Autodesk Fusion 360 part; units mm, degrees
sketch "Sketch1" plane through (0, 0, 0) normal (0, 1, 0) x (1, 0, 0) in component "Raam_v3"
  line L0 (-100, 100) -> (100, 100)
  line L1 (100, 100) -> (100, -100)
  line L2 (100, -100) -> (-100, -100)
  line L3 (-100, -100) -> (-100, 100)
  circle A0 centre (0, 0) radius 82.5
  line L4 (-70.5, -70.5) -> (70.5, -70.5) construction
  line L5 (70.5, -70.5) -> (70.5, 70.5) construction
  line L6 (70.5, 70.5) -> (-70.5, 70.5) construction
  line L7 (-70.5, 70.5) -> (-70.5, -70.5) construction
  line L8 (-46, -100) -> (46, -100)
  line L9 (46, -100) -> (46, -68)
  line L10 (46, -68) -> (-46, -68)
  line L11 (-46, -68) -> (-46, -100)
  line L12 (-46, 100) -> (46, 100)
  line L13 (46, 100) -> (46, 68)
  line L14 (46, 68) -> (-46, 68)
  line L15 (-46, 68) -> (-46, 100)
  circle A1 centre (70.5, -70.5) radius 5
  circle A2 centre (-70.5, -70.5) radius 5
  circle A3 centre (70.5, 70.5) radius 5
  circle A4 centre (-70.5, 70.5) radius 5
  line L16 (-91.25, -91.25) -> (91.25, -91.25) construction
  line L17 (91.25, -91.25) -> (91.25, 91.25) construction
  line L18 (91.25, 91.25) -> (-91.25, 91.25) construction
  line L19 (-91.25, 91.25) -> (-91.25, -91.25) construction
  line L20 (0, -100) -> (0, 100) construction
  line L21 (-100, 0) -> (100, 0) construction
  line L22 (-100, -75) -> (-74.4285, -100)
  line L23 (100, -75) -> (75.5588, -100)
  line L24 (-100, 75) -> (-75.5588, 100)
  line L25 (74.4285, 100) -> (100, 75)
  circle A5 centre (-91.25, 0) radius 1.5
  circle A6 centre (91.25, 0) radius 1.5
  line L26 (-100, -75) -> (100, -75) construction
  circle A7 centre (91.25, -75) radius 1.5
  line L27 (-100, 75) -> (100, 75) construction
  circle A8 centre (91.25, 75) radius 1.5
  circle A9 centre (-91.25, 75) radius 1.5
  circle A10 centre (-91.25, -75) radius 1.5
  line L28 (-95.1383, -79.753) -> (-77.6201, -79.753)
  line L29 (-77.6201, -79.753) -> (-77.6201, -96.8797)
  line L30 (-83.7274, -79.753) -> (-83.7274, -80)
  line L31 (95.3116, -79.7956) -> (78.4368, -79.7956)
  line L32 (78.4368, -79.7956) -> (78.4368, -97.0562)
  line L33 (-95.1178, 79.9938) -> (-80.1166, 79.9938)
  line L34 (-80.1166, 79.9938) -> (-80.1166, 95.3379)
  line L35 (94.9708, 79.9168) -> (79.5428, 79.9168)
  line L36 (79.5428, 79.9168) -> (79.5428, 95)
  dimension "d1" = 200
  dimension "d2" = 200
  dimension "d3" = 165
  dimension "d6" = 141
  dimension "d7" = 141
  dimension "d8" = 29.5
  dimension "d9" = 29.5
  dimension "d11" = 100
  dimension "d12" = 100
  dimension "d18" = 92
  dimension "d19" = 32
  dimension "d20" = 46
  dimension "d21" = 92
  dimension "d22" = 32
  dimension "d23" = 46
  dimension "d24" = 10
  dimension "d25" = 10
  dimension "d26" = 10
  dimension "d27" = 10
  dimension "d28" = 182.5
  dimension "d29" = 182.5
  dimension "d30" = 70.5
  dimension "d31" = 8.75
  dimension "d32" = 8.75
  dimension "d33" = 3
  dimension "d34" = 3
  dimension "d53" = 12.3744
  dimension "d54" = 12.3744
  dimension "d55" = 12.3744
  dimension "d56" = 12.3744
  dimension "d57" = 41.7193
  dimension "d58" = 41.7193
  dimension "d59" = 75
  dimension "d60" = 3
  dimension "d61" = 75
  dimension "d62" = 3
  dimension "d63" = 3
  dimension "d64" = 3
extrude "Extrude11" add sketch "Sketch1" along normal blind 1.25 contours L0 A0 L12 L13 L15 | L2 A0 L8 L9 L11 makes body 1 at (0, 0, -94.1667) makes body 2 at (0, 0, 94.1667) in component "Raam_v3"
extrude "Extrude10" add sketch "Sketch1" along normal blind 2 separate body contours L0 L2 L3 A0 L11 L15 L22 L24 L28 L29 L33 L34 | L0 L1 L2 A0 L9 L13 L23 L25 L31 L32 L35 L36 makes body 3 at (-63.4107, 0, -91.7181) makes body 4 at (63.4107, 2, 91.7181) in component "Raam_v3"
extrude "Extrude12" add sketch "Sketch1" along normal blind 3.5 contours A2 bodies 3 in component "Raam_v3"
extrude "Extrude13" add sketch "Sketch1" along normal blind 3.5 contours A1 bodies 4 in component "Raam_v3"
extrude "Extrude14" add sketch "Sketch1" along normal blind 3.5 contours A4 bodies 3 in component "Raam_v3"
extrude "Extrude15" add sketch "Sketch1" along normal blind 3.5 contours A3 bodies 4 in component "Raam_v3"
extrude "Extrude16" add 1 faces at (63.4107, 2, 91.7181) along direction (0, 1, 0) blind 2 on bodies 4 bodies 4 in component "Raam_v3"
extrude "Extrude17" add 1 faces at (-63.4107, 2, -91.7181) along direction (0, 1, 0) blind 2 on bodies 3 bodies 3 in component "Raam_v3"
extrude "Extrude18" add 1 faces at (0, 1.25, 94.1667) along direction (0, 1, 0) blind 1 on bodies 2 bodies 2 3 4 in component "Raam_v3"
extrude "Extrude19" add 1 faces at (0, 1.25, -94.1667) along direction (0, 1, 0) blind 1 on bodies 1 bodies 1 2 in component "Raam_v3"
extrude "Extrude20" add 1 faces at (-69.0538, 3.5, 70.0197) along direction (0, 1, 0) blind 4 on bodies 1 bodies 1 in component "Raam_v3"
extrude "Extrude21" cut 1 faces at (-69.0538, 7.5, 70.0197) along direction (0, -1, 0) blind 1 on bodies 1 bodies 1 in component "Raam_v3"
extrude "Extrude22" add 1 faces at (71.8216, 3.5, 69.804) along direction (0, 1, 0) blind 3 on bodies 1 bodies 1 in component "Raam_v3"
extrude "Extrude23" add 1 faces at (-69.0538, 3.5, -70.9803) along direction (0, 1, 0) blind 3 on bodies 1 bodies 1 in component "Raam_v3"
extrude "Extrude24" cut 1 faces at (-63.4107, 4, -91.7181) along direction (0, -1, 0) blind 1 on bodies 1 bodies 1 in component "Raam_v3"
extrude "Extrude25" cut 1 faces at (63.4107, 4, 91.7181) along direction (0, -1, 0) blind 1 on bodies 1 bodies 1 in component "Raam_v3"
extrude "Extrude26" cut 1 faces at (0, 2.25, 94.1667) along direction (0, -1, 0) blind 0.5 on bodies 1 bodies 1 in component "Raam_v3"
extrude "Extrude27" cut 1 faces at (0, 2.25, -94.1667) along direction (0, -1, 0) blind 0.5 on bodies 1 bodies 1 in component "Raam_v3"
extrude "Extrude28" cut 1 faces at (-69.0538, 6.5, 70.0197) along direction (0, -1, 0) blind 1 on bodies 1 bodies 1 in component "Raam_v3"
extrude "Extrude29" cut 1 faces at (71.8216, 6.5, 69.804) along direction (0, -1, 0) blind 1 on bodies 1 bodies 1 in component "Raam_v3"
extrude "Extrude30" cut 1 faces at (71.8216, 3.5, -71.196) along direction (0, -1, 0) blind 1 on bodies 1 bodies 1 in component "Raam_v3"
extrude "Extrude31" cut 1 faces at (-69.0538, 6.5, -70.9803) along direction (0, -1, 0) blind 1 on bodies 1 bodies 1 in component "Raam_v3"
extrude "Extrude32" add 1 faces at (71.8216, 2.5, -71.196) along direction (0, 1, 0) blind 3 on bodies 1 bodies 1 in component "Raam_v3"
extrude "Extrude2" [suppressed] in component "Raam_v3"
extrude "Extrude1" [suppressed] in component "Raam_v3"
extrude "Extrude3" [suppressed] in component "Raam_v3"
extrude "Extrude4" [suppressed] in component "Raam_v3"
extrude "Extrude5" [suppressed] in component "Raam_v3"
extrude "Extrude6" [suppressed] in component "Raam_v3"
extrude "Extrude7" [suppressed] in component "Raam_v3"
extrude "Extrude8" [suppressed] in component "Raam_v3"
extrude "Extrude9" [suppressed] in component "Raam_v3"
hole "Hole1" [suppressed] in component "Raam_v3"
hole "Hole2" [suppressed] in component "Raam_v3"
hole "Hole3" [suppressed] in component "Raam_v3"
move_body "Move1" [suppressed] in component "Raam_v3"
move_body "Move2" [suppressed] in component "Raam_v3"
hole "Hole4" [suppressed] in component "Raam_v3"
delete_face "DeleteFace1" [suppressed] in component "Raam_v3"
delete_face "DeleteFace2" [suppressed] in component "Raam_v3"
hole "Hole5" [suppressed] in component "Raam_v3"
delete_face "DeleteFace3" [suppressed] in component "Raam_v3"
hole "Hole6" [suppressed] in component "Raam_v3"
hole "Hole7" [suppressed] in component "Raam_v3"
component "Raam_v3" placed x (1, 0, 0) y (0, 1, 0) z (0, 0, 1) at (0, 0, 0)
CAD build for the part. Positions are in the model's coordinates, mm. A direction names the side the tool comes from. Round coordinates to 2 decimals unless told otherwise and drop trailing zeros. Write each loop counter-clockwise with the first axis right and the second up, starting at its lowest first coordinate (ties: lowest second). Pieces come first, ordered by that corner, then holes. Notation, with made-up numbers: (-5, -36) - (41, -36) arc R13 cw to (41, -19) - close; hole circle Ø10 at (-19, -3). An arc over 180 degrees is marked (long way). Return JSON: item names as keys, results as strings. Group by question number.
Item 1: Band-saw the part on C-C on y = 4.65. List the corners of the cut face in (x, z).
Item 2: Band-saw the part on B-B on x = 23. List the corners of the cut face in (y, z), plus the area to 3 significant figures.
Item 3: Mould opens along Z. For faces 4 (the face through (-97.603, 1.479, 77.343)), 5 (the face through (-71, 5.5, -71)), 6 (the face through (75.119, 4.232, 68.585)) say: +Z half, -Z half, draft (parallel to the pull), parting line (faces both ways), or undercut.
Item 4: Band-saw the part on A-A on z = -14.5. List the corners of the cut face in (x, y).
Item 5: 3-axis set-ups, long thin cutter, end or side, ignore diameter. For faces 1 (the face through (-1, 1.75, 88)), 2 (the face through (75.27, 4.23, -69)), 3 (the face through (97.45, 1.479, -77.493)): which of +Z, -Z, +X, -X, +Y, -Y reach the whole face in a straight line?
Item 6: Band-saw the part on D-D on x = -70.5. List the corners of the cut face in (y, z).
Item 7: Probe probe 1 along Z at (x, y) = (-91.25, 0.95); probe 2 along X at (y, z) = (1.45, 0); probe 3 along Z at (x, y) = (-90, 1.6). List the from-to ranges inside material, lowest first.
Item 8: Flat gauge pins, fed straight in: pin 1 Ø1.5 at (x, y) = (0, 4) entering from -Z; pin 2 Ø1 at (y, z) = (2, 86) entering from +X; pin 3 Ø1.4 at (y, z) = (2.5, -88.5) entering from +X; pin 4 Ø1.5 at (y, z) = (2, 87.5) entering from -X. Where does each tip first touch, or does it go through?
Resolved:
{
 "1": {"outline": "circle Ø10 at (-70.5, -70.5); circle Ø10 at (-70.5, 70.5); circle Ø10 at (70.5, -70.5); circle Ø10 at (70.5, 70.5)"},
 "2": {"outline": "(0, -100) - (1.75, -100) - (1.75, -79.23) - (0, -79.23) - close; (0, 79.23) - (1.75, 79.23) - (1.75, 100) - (0, 100) - close", "area": "72.7 mm²"},
 "3": {"face 4": "+Z half", "face 5": "draft", "face 6": "undercut"},
 "4": {"outline": "(-100, 0) - (-81.22, 0) - (-81.22, 3) - (-100, 3) - close; (81.22, 0) - (100, 0) - (100, 3) - (81.22, 3) - close"},
 "5": {"face 1": "+Z, -Z, +Y", "face 2": "+Y", "face 3": "-Z, +X, +Y, -Y"},
 "6": {"outline": "(0, -100) - (3, -100) - (3, -75.5) - (5.5, -75.5) - (5.5, -65.5) - (3, -65.5) - (3, -42.85) - (0, -42.85) - close; (0, 42.85) - (3, 42.85) - (3, 65.5) - (5.5, 65.5) - (5.5, 75.5) - (3, 75.5) - (3, 100) - (0, 100) - close"},
 "7": {"probe 1": "z = -79.99 to -76.5, -73.5 to -1.5, 1.5 to 73.5, 76.5 to 79.75", "probe 2": "x = -100 to -92.75, -89.75 to -82.5, 82.5 to 89.75, 92.75 to 100", "probe 3": "z = -79.99 to -75.83, -74.17 to -0.83, 0.83 to 74.17, 75.83 to 79.75"},
 "8": {"pin 1": "passes through", "pin 2": "stops at x = 78.44", "pin 3": "stops at x = 79.54", "pin 4": "stops at x = -77.62"}
}
